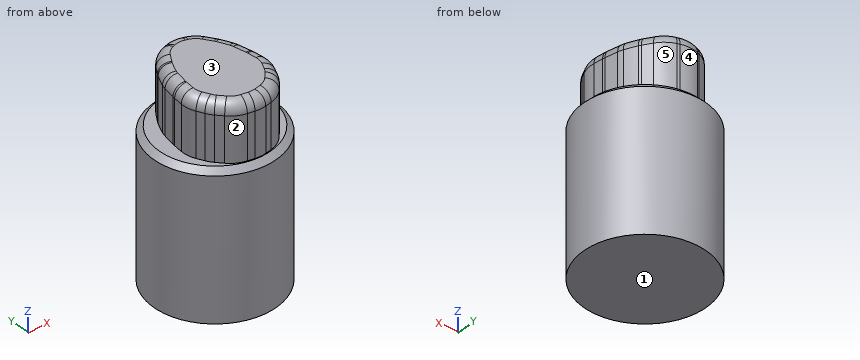
```python
from build123d import *

# Parameters (mm, degrees)
F2_DEPTH = 36
F3_R     = 2
F4_R     = 11
F5_DEPTH = 26
F6_SIZE  = 1


with BuildPart() as f2:
    # F1 (on Top) → F2 (new body)
    with BuildSketch(Plane.XY):
        with BuildLine():
            Line((1.982116, 9.333126), (1.594405, 9.46357))
            ThreePointArc((1.594405, 9.46357), (0, 9.724596), (-1.594405, 9.46357))
            Line((-1.594405, 9.46357), (-1.982116, 9.333126))
            ThreePointArc((-1.982116, 9.333126), (-3.454217, 8.543398), (-4.584004, 7.312814))
            Line((-4.584004, 7.312814), (-5.540871, 5.835876))
            ThreePointArc((-5.540871, 5.835876), (-5.659922, 5.642646), (-5.770081, 5.444212))
            ThreePointArc((-5.770081, 5.444212), (-6.285484, 4.401197), (-6.747831, 3.333603))
            ThreePointArc((-6.747831, 3.333603), (-6.902422, 2.892031), (-7.015063, 2.437942))
            Line((-7.015063, 2.437942), (-7.456926, 0.216547))
            ThreePointArc((-7.456926, 0.216547), (-7.495184, -0.000739), (-7.523819, -0.2195))
            Line((-7.523819, -0.2195), (-7.702549, -1.866568))
            ThreePointArc((-7.702549, -1.866568), (-7.661217, -3.220061), (-7.251011, -4.510557))
            Line((-7.251011, -4.510557), (-6.664507, -5.735999))
            ThreePointArc((-6.664507, -5.735999), (-6.323741, -6.337337), (-5.903302, -6.885936))
            Line((-5.903302, -6.885936), (-4.94414, -7.972769))
            ThreePointArc((-4.94414, -7.972769), (-3.688499, -8.998323), (-2.170731, -9.568215))
            Line((-2.170731, -9.568215), (-0.975452, -9.805971))
            ThreePointArc((-0.975452, -9.805971), (0, -9.902044), (0.975452, -9.805971))
            Line((0.975452, -9.805971), (2.170731, -9.568215))
            ThreePointArc((2.170731, -9.568215), (3.688499, -8.998323), (4.94414, -7.972769))
            Line((4.94414, -7.972769), (5.903302, -6.885936))
            ThreePointArc((5.903302, -6.885936), (6.323741, -6.337337), (6.664507, -5.735999))
            Line((6.664507, -5.735999), (7.251011, -4.510557))
            ThreePointArc((7.251011, -4.510557), (7.661217, -3.220061), (7.702549, -1.866568))
            Line((7.702549, -1.866568), (7.523819, -0.2195))
            ThreePointArc((7.523819, -0.2195), (7.495184, -0.000739), (7.456926, 0.216547))
            Line((7.456926, 0.216547), (7.015063, 2.437942))
            ThreePointArc((7.015063, 2.437942), (6.902422, 2.892031), (6.747831, 3.333603))
            ThreePointArc((6.747831, 3.333603), (6.285484, 4.401197), (5.770081, 5.444212))
            ThreePointArc((5.770081, 5.444212), (5.659922, 5.642646), (5.540871, 5.835876))
            Line((5.540871, 5.835876), (4.584004, 7.312814))
            ThreePointArc((4.584004, 7.312814), (3.454217, 8.543398), (1.982116, 9.333126))
        make_face()
    extrude(amount=F2_DEPTH)

    # F3
    f3_edges = [f2.edges().sort_by_distance(p)[0] for p in [
        (3.688499, -8.998323, 36),
    ]]
    fillet(f3_edges, radius=F3_R)

    # F4 (on face) → F5 (join)
    with BuildSketch(Plane(origin=(0, 0, 0), x_dir=(1, 0, 0), z_dir=(0, 0, -1))):
        Circle(F4_R)
        with BuildLine():
            ThreePointArc((-7.702549, 1.866568), (-7.661217, 3.220061), (-7.251011, 4.510557))
            Line((-7.251011, 4.510557), (-6.664507, 5.735999))
            ThreePointArc((-6.664507, 5.735999), (-6.323741, 6.337337), (-5.903302, 6.885936))
            Line((-5.903302, 6.885936), (-4.94414, 7.972769))
            ThreePointArc((-4.94414, 7.972769), (-3.688499, 8.998323), (-2.170731, 9.568215))
            Line((-2.170731, 9.568215), (-0.975452, 9.805971))
            ThreePointArc((-0.975452, 9.805971), (0, 9.902044), (0.975452, 9.805971))
            Line((0.975452, 9.805971), (2.170731, 9.568215))
            ThreePointArc((2.170731, 9.568215), (3.688499, 8.998323), (4.94414, 7.972769))
            Line((4.94414, 7.972769), (5.903302, 6.885936))
            ThreePointArc((5.903302, 6.885936), (6.323741, 6.337337), (6.664507, 5.735999))
            Line((6.664507, 5.735999), (7.251011, 4.510557))
            ThreePointArc((7.251011, 4.510557), (7.661217, 3.220061), (7.702549, 1.866568))
            Line((7.702549, 1.866568), (7.523819, 0.2195))
            ThreePointArc((7.523819, 0.2195), (7.495184, 0.000739), (7.456926, -0.216547))
            Line((7.456926, -0.216547), (7.015063, -2.437942))
            ThreePointArc((7.015063, -2.437942), (6.902422, -2.892031), (6.747831, -3.333603))
            ThreePointArc((6.747831, -3.333603), (6.285484, -4.401197), (5.770081, -5.444212))
            ThreePointArc((5.770081, -5.444212), (5.659922, -5.642646), (5.540871, -5.835876))
            Line((5.540871, -5.835876), (4.584004, -7.312814))
            ThreePointArc((4.584004, -7.312814), (3.454217, -8.543398), (1.982116, -9.333126))
            Line((1.982116, -9.333126), (1.594405, -9.46357))
            ThreePointArc((1.594405, -9.46357), (0, -9.724596), (-1.594405, -9.46357))
            Line((-1.594405, -9.46357), (-1.982116, -9.333126))
            ThreePointArc((-1.982116, -9.333126), (-3.454217, -8.543398), (-4.584004, -7.312814))
            Line((-4.584004, -7.312814), (-5.540871, -5.835876))
            ThreePointArc((-5.540871, -5.835876), (-5.659922, -5.642646), (-5.770081, -5.444212))
            ThreePointArc((-5.770081, -5.444212), (-6.285484, -4.401197), (-6.747831, -3.333603))
            ThreePointArc((-6.747831, -3.333603), (-6.902422, -2.892031), (-7.015063, -2.437942))
            Line((-7.015063, -2.437942), (-7.456926, -0.216547))
            ThreePointArc((-7.456926, -0.216547), (-7.495184, 0.000739), (-7.523819, 0.2195))
            Line((-7.523819, 0.2195), (-7.702549, 1.866568))
        make_face(mode=Mode.SUBTRACT)
    extrude(amount=-F5_DEPTH)

    # F6
    f6_edges = [f2.edges().sort_by_distance(p)[0] for p in [
        (-11, 0, 26),
    ]]
    chamfer(f6_edges, length=F6_SIZE)


solid = f2.part
```
Work out the finished part from the listing and answer in its coordinate system (mm). Face numbers are marked on the shaded views. A direction names the side the tool comes from. Round coordinates to 2 decimals unless told otherwise and drop trailing zeros. Order: outer loops, then holes, each group sorted by start corner. A loop starts at its lowest first (then second) coordinate and runs counter-clockwise, first axis right, second up.
Q1. Given pin 1 Ø2 at (x, z) = (-7.5, 8) entering from -Y; pin 2 Ø12 at (y, z) = (6, 31.5) entering from +X; pin 3 Ø5 at (y, z) = (-9, 21) entering from -X, each flat-ended and moving along its own axis, determine where each tip first touches the part or whether it passes through.
Solution:
pin 1: stops at y = -8.87
pin 2: stops at x = 9.34
pin 3: stops at x = -8.87
Q2. A tool of negligible diameter and unlimited length cuts with its end or side. For the marked faces 1, 2, 3, 4 and 5, from which of +Z, -Z, +X, -X, +Y, -Y can it reach the whole face along a straight path? Write none if from no direction.
Solution:
face 1: -Z, +X, -X, +Y, -Y
face 2: +Z, -X, -Y
face 3: +Z, +X, -X, +Y, -Y
face 4: +Z, +Y
face 5: +Z, +X, +Y
Q3. A cutting plane is placed at A-A, the plane x = 0. Determine the outline of the cut face in (y, z), then the cut area to 3 significant figures.
Solution:
outline: (-11, 0) - (11, 0) - (11, 25) - (10, 26) - (9.72, 26) - (9.72, 34) arc R2 ccw to (7.72, 36) - (-7.9, 36) arc R2 ccw to (-9.9, 34) - (-9.9, 26) - (-10, 26) - (-11, 25) - close
area: 766 mm2
Q4. A cutting plane is placed at C-C, the plane z = 23.5. Determine the outline of the cut face in (x, y), then the cut area to 3 significant figures.
Solution:
outline: circle Ø22 at (0, 0)
area: 380 mm2
Q5. Find the intervals of material crossed by line 1 along Z through (x, y) = (5.25, -4.5); line 2 along Z through (x, y) = (-8.75, 0); line 3 along Y through (x, z) = (-0.25, 4.5), in increasing order.
Solution:
line 1: z = 0 to 35.99
line 2: z = 0 to 26
line 3: y = -11 to 11
